The listing builds one solid part. Answer for the finished solid, in the listing's coordinates (mm). A direction names the side the tool comes from. Coordinates: 2 decimals unless noted, no trailing zeros. Loops run counter-clockwise (first coordinate to the right, second up) from the corner with the lowest first, then second, coordinate; pieces in that order, holes last. Notation, with made-up numbers: (8.5, 85) - (17.5, 85) arc R28 cw to (17.5, 111) - close; hole circle Ø5 at (30.25, 78). An arc over 180 degrees is marked (long way). Write each question's results on one line, items separated by ' | '. Start each with the question number.
(1) Find section A-A on z = -30. Determine the outline of the cut face in (x, y), then the cut area to 3 significant figures.
(2) Find section C-C on x = 3. Determine the outline of the cut face in (y, z).
(3) Consider line 1 (Y direction, x = 22.5, z = -151); line 2 (Y direction, x = 2.15, z = -30); line 3 (Y direction, x = 2, z = -42). Determine where each line is inside the solid, lowest interval first. Write a range as from..to.
(4) Find section D-D on x = 22. Determine the outline of the cut face in (y, z), then the cut area to 3 significant figures.
(5) Find section B-B on y = -12.5. Determine the outline of the cut face in (x, z), then the cut area to 3 significant figures.
(6) Given pin 1 Ø1.5 at (x, z) = (3.5, -139.5) entering from +Y; pin 2 Ø13 at (y, z) = (15.5, -42.5) entering from +X; pin 3 Ø5 at (x, y) = (21.5, -19) entering from +Z, each flat-ended and moving along its own axis, determine where each tip first touches the part or whether it passes through.
(7) Determine the mould class of faces 1 (the cylindrical face through (2.54, 15.57, -28.5)), 2 (the flat face through (20, 0, -155)), 3 (the flat face through (4, -25, -95)) for opening direction Y: released by +Y, released by -Y, zero draft, split by the parting line, or undercut.
(8) For faces 4 (the flat face through (20, 25, -152)), 5 (the flat face through (3, 20, -125)), 6 (the flat face through (5, 0, -74)), determine the directions among +Z, -Z, +X, -X, +Y, -Y from which every point of the face is accessible in a straight line to the end or side of a thin tool.
from build123d import *

# Parameters (mm, degrees)
BOSS_EXTRUDE5_DEPTH = 25
CUT_EXTRUDE2_REACH  = 162.857
SKETCH6_R           = 1.5
SKETCH6_R_2         = 2.5
SKETCH6_R_3         = 4
SKETCH6_W           = 20
SKETCH6_H           = 10
CUT_EXTRUDE3_REACH  = 159.242
SKETCH7_R           = 2.5


with BuildPart() as part:
    # Sketch4 → Boss-Extrude5 (new, symmetric)
    with BuildSketch(Plane(origin=(0, 0, 0), x_dir=(1, 0, 0), z_dir=(0, 1, 0))):
        Polygon((0, 0), (5, 0), (5, 150), (40, 150), (40, 155), (0, 155), align=None)
    extrude(amount=BOSS_EXTRUDE5_DEPTH, both=True)

    # Sketch6 → Cut-Extrude2 (cut, up to next)
    with BuildSketch(Plane(origin=(5, 0, 0), x_dir=(0, 0, -1), z_dir=(1, 0, 0)), mode=Mode.PRIVATE) as cut_extrude2_sk1:
        with Locations((5, 15.5)):
            Circle(SKETCH6_R)
    cut_extrude2_tool1 = extrude(cut_extrude2_sk1.sketch, amount=-CUT_EXTRUDE2_REACH, mode=Mode.PRIVATE) & part.part
    # Sketch6 → Cut-Extrude2 (cut, up to next)
    with BuildSketch(Plane(origin=(5, 0, 0), x_dir=(0, 0, -1), z_dir=(1, 0, 0)), mode=Mode.PRIVATE) as cut_extrude2_sk2:
        with Locations((17.5, 15.5)):
            Circle(SKETCH6_R_2)
    cut_extrude2_tool2 = extrude(cut_extrude2_sk2.sketch, amount=-CUT_EXTRUDE2_REACH, mode=Mode.PRIVATE) & part.part
    # Sketch6 → Cut-Extrude2 (cut, up to next)
    with BuildSketch(Plane(origin=(5, 0, 0), x_dir=(0, 0, -1), z_dir=(1, 0, 0)), mode=Mode.PRIVATE) as cut_extrude2_sk3:
        with Locations((30, 15.5)):
            Circle(SKETCH6_R)
    cut_extrude2_tool3 = extrude(cut_extrude2_sk3.sketch, amount=-CUT_EXTRUDE2_REACH, mode=Mode.PRIVATE) & part.part
    # Sketch6 → Cut-Extrude2 (cut, up to next)
    with BuildSketch(Plane(origin=(5, 0, 0), x_dir=(0, 0, -1), z_dir=(1, 0, 0)), mode=Mode.PRIVATE) as cut_extrude2_sk4:
        with Locations((42.5, 15.5)):
            Circle(SKETCH6_R_3)
    cut_extrude2_tool4 = extrude(cut_extrude2_sk4.sketch, amount=-CUT_EXTRUDE2_REACH, mode=Mode.PRIVATE) & part.part
    # Sketch6 → Cut-Extrude2 (cut, up to next)
    with BuildSketch(Plane(origin=(5, 0, 0), x_dir=(0, 0, -1), z_dir=(1, 0, 0)), mode=Mode.PRIVATE) as cut_extrude2_sk5:
        with Locations((135, 20)):
            Rectangle(SKETCH6_W, SKETCH6_H)
    cut_extrude2_tool5 = extrude(cut_extrude2_sk5.sketch, amount=-CUT_EXTRUDE2_REACH, mode=Mode.PRIVATE) & part.part
    add(cut_extrude2_tool1.solids().sort_by_distance((5, 15.5, -5))[0], mode=Mode.SUBTRACT)
    add(cut_extrude2_tool2.solids().sort_by_distance((5, 15.5, -17.5))[0], mode=Mode.SUBTRACT)
    add(cut_extrude2_tool3.solids().sort_by_distance((5, 15.5, -30))[0], mode=Mode.SUBTRACT)
    add(cut_extrude2_tool4.solids().sort_by_distance((5, 15.5, -42.5))[0], mode=Mode.SUBTRACT)
    add(cut_extrude2_tool5.solids().sort_by_distance((5, 20, -135))[0], mode=Mode.SUBTRACT)

    # Sketch7 → Cut-Extrude3 (cut, up to next)
    with BuildSketch(Plane.XY.offset(-150), mode=Mode.PRIVATE) as cut_extrude3_sk1:
        with Locations((22.5, 12.5)):
            Circle(SKETCH7_R)
    cut_extrude3_tool1 = extrude(cut_extrude3_sk1.sketch, amount=-CUT_EXTRUDE3_REACH, mode=Mode.PRIVATE) & part.part
    # Sketch7 → Cut-Extrude3 (cut, up to next)
    with BuildSketch(Plane.XY.offset(-150), mode=Mode.PRIVATE) as cut_extrude3_sk2:
        with Locations((22.5, -12.5)):
            Circle(SKETCH7_R)
    cut_extrude3_tool2 = extrude(cut_extrude3_sk2.sketch, amount=-CUT_EXTRUDE3_REACH, mode=Mode.PRIVATE) & part.part
    add(cut_extrude3_tool1.solids().sort_by_distance((22.5, 12.5, -150))[0], mode=Mode.SUBTRACT)
    add(cut_extrude3_tool2.solids().sort_by_distance((22.5, -12.5, -150))[0], mode=Mode.SUBTRACT)


solid = part.part
Values:
1) outline: (0, -25) - (5, -25) - (5, 14) - (0, 14) - close; (0, 17) - (5, 17) - (5, 25) - (0, 25) - close | area: 235 mm²
2) outline: (-25, -155) - (25, -155) - (25, -145) - (15, -145) - (15, -125) - (25, -125) - (25, 0) - (-25, 0) - close; hole circle Ø8 at (15.5, -42.5); hole circle Ø5 at (15.5, -17.5); hole circle Ø3 at (15.5, -30); hole circle Ø3 at (15.5, -5)
3) line 1: y = -25..-15, -10..10, 15..25 | line 2: y = -25..14, 17..25 | line 3: y = -25..11.53, 19.47..25
4) outline: (-25, -155) - (-14.95, -155) - (-14.95, -150) - (-25, -150) - close; (-10.05, -155) - (10.05, -155) - (10.05, -150) - (-10.05, -150) - close; (14.95, -155) - (25, -155) - (25, -150) - (14.95, -150) - close | area: 201 mm²
5) outline: (0, -155) - (20, -155) - (20, -150) - (5, -150) - (5, 0) - (0, 0) - close; (25, -155) - (40, -155) - (40, -150) - (25, -150) - close | area: 925 mm²
6) pin 1: stops at y = 15 | pin 2: stops at x = 5 | pin 3: stops at z = -150
7) face 1: undercut | face 2: zero draft | face 3: released by -Y
8) face 4: +Z, -Z, +X, -X, +Y | face 5: +X, -X, +Y | face 6: +Z, +X, +Y, -Y
